Input: part model. Units: mm. Frame: model coordinates. Face numbers are marked on the shaded views. A direction names the side the tool comes from. Coordinates: 2 decimals unless noted, no trailing zeros. Loops run counter-clockwise (first coordinate to the right, second up) from the corner with the lowest first, then second, coordinate; pieces in that order, holes last.
Item 1: Section D-D on x = 114.5. Return loops of the section in (y, z), and give its area (3 significant figures).
Item 2: Section C-C on z = 19. Return loops of the section in (x, y).
Item 3: Section A-A on y = 160. Return loops of the section in (x, z), and give its area (3 significant figures).
Item 4: Section B-B on x = -44.5. Return loops of the section in (y, z), and give its area (3 significant figures).
Item 5: Ray query, line 1 along Y through (x, z) = (-106, 48); line 2 along X through (y, z) = (115.5, 12); line 3 along Z through (x, y) = (-24.5, 182.5). Return the intervals inside material, ascending.
Item 6: Reachability of the marked faces 5 and 6 from +Z, -Z, +X, -X, +Y, -Y: full face, straight path, thin tool, end or side. Return the list, or none.
Item 7: Pull-direction query (X, two-part tool) for the marked faces 1, 2, 3 and 4; classes: released by +X, released by -X, zero draft, split by the parting line, or undercut.
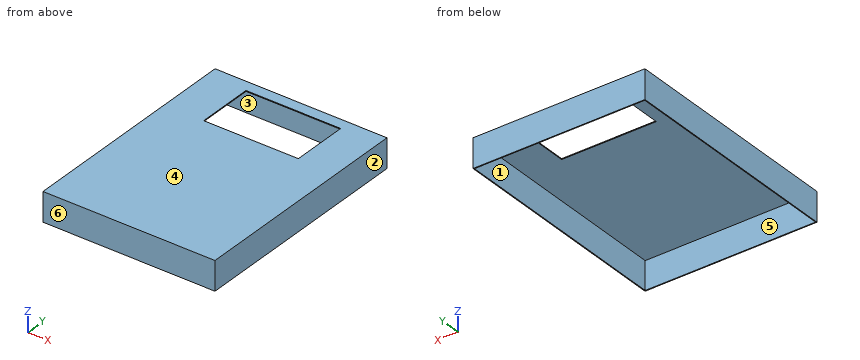
```python
from build123d import *

# Parameters (mm, degrees)
SKETCH1_W           = 300
SKETCH1_H           = 400
BOSS_EXTRUDE1_DEPTH = 50.8
SHELL1_T            = -1.500000048
SKETCH2_W           = 165.1
SKETCH2_H           = 98.425
CUT_EXTRUDE1_DEPTH  = 256.109074711


with BuildPart() as part:
    # Sketch1 → Boss-Extrude1 (new body)
    with BuildSketch(Plane.XY):
        Rectangle(SKETCH1_W, SKETCH1_H)
    extrude(amount=BOSS_EXTRUDE1_DEPTH)

    # Shell1
    shell1_openings = [part.faces().sort_by_distance(p)[0] for p in [
        (0, 0, 0),
    ]]
    offset(amount=SHELL1_T, openings=shell1_openings, kind=Kind.INTERSECTION)

    # Sketch2 → Cut-Extrude1 (cut, through all)
    with BuildSketch(Plane.XY.offset(50.8)):
        with Locations((1.151083914, 131.430868262)):
            Rectangle(SKETCH2_W, SKETCH2_H)
    extrude(amount=-CUT_EXTRUDE1_DEPTH, mode=Mode.SUBTRACT)


solid = part.part
```
Results found:
1. outline: (-200, 0) - (-198.5, 0) - (-198.5, 49.3) - (198.5, 49.3) - (198.5, 0) - (200, 0) - (200, 50.8) - (-200, 50.8) - close
1. area: 748 mm2
2. outline: (-150, -200) - (150, -200) - (150, 200) - (-150, 200) - close; hole (-148.5, -198.5) - (148.5, -198.5) - (148.5, 198.5) - (-148.5, 198.5) - close
3. outline: (-150, 0) - (-148.5, 0) - (-148.5, 49.3) - (-81.4, 49.3) - (-81.4, 50.8) - (-150, 50.8) - close; (83.7, 49.3) - (148.5, 49.3) - (148.5, 0) - (150, 0) - (150, 50.8) - (83.7, 50.8) - close
3. area: 350 mm2
4. outline: (-200, 0) - (-198.5, 0) - (-198.5, 49.3) - (82.22, 49.3) - (82.22, 50.8) - (-200, 50.8) - close; (180.64, 49.3) - (198.5, 49.3) - (198.5, 0) - (200, 0) - (200, 50.8) - (180.64, 50.8) - close
4. area: 600 mm2
5. line 1: y = -200 to -198.5, 198.5 to 200
5. line 2: x = -150 to -148.5, 148.5 to 150
5. line 3: z = 49.3 to 50.8
6. face 5: -Z
6. face 6: +Z, -Z, +X, -X, -Y
7. face 1: undercut
7. face 2: released by +X
7. face 3: undercut
7. face 4: zero draft
